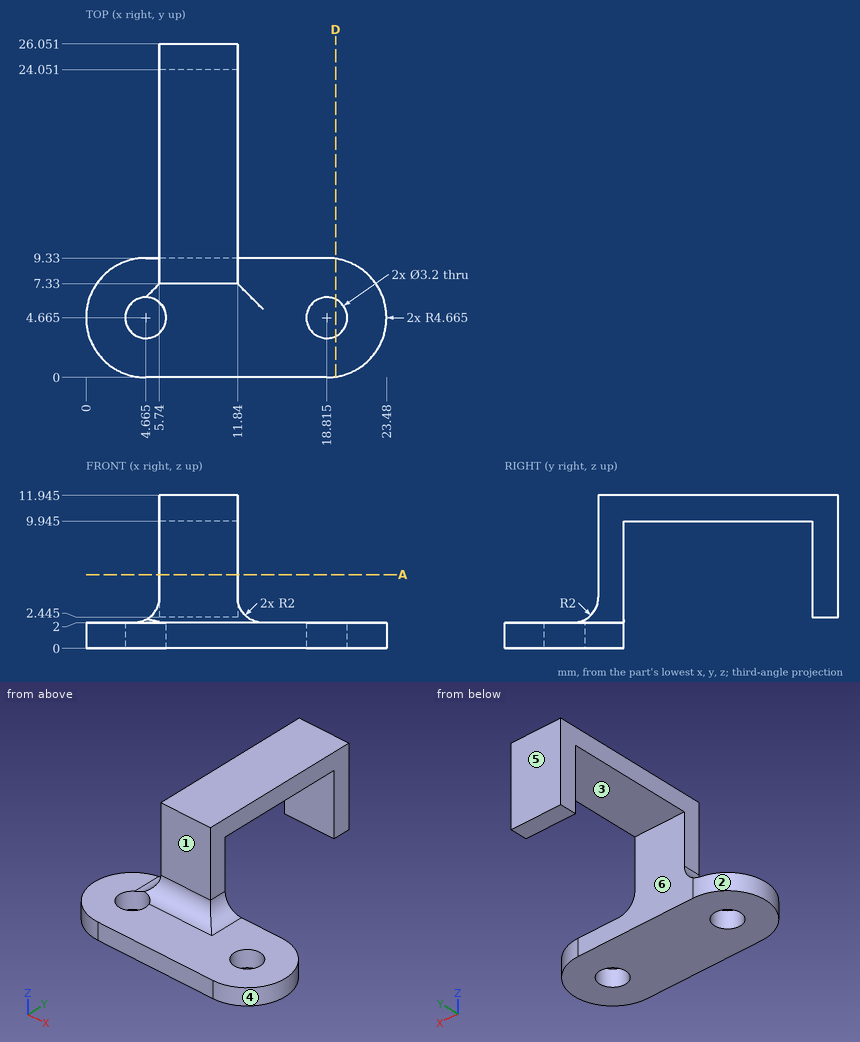
The drawing under review shows one solid part. Ordinate dimensions are in mm from its lowest x, y, z. A direction names the side the tool comes from. Give positions to 0.01 mm unless a question says otherwise; leave off trailing zeros. Write each loop counter-clockwise with the first axis right and the second up, starting at its lowest first coordinate (ties: lowest second). Pieces come first, ordered by that corner, then holes. Notation, with made-up numbers: (28, 42) -> (59, 42) arc R26 cw to (59, 62) -> close; hole circle Ø10 at (-17.75, 86). An arc over 180 degrees is marked (long way). Put each result on its own line as item: value.
(1) We need section D-D, the plane x = 19.5. Give the boundary of the cut face in (y, z), and give its area (3 significant figures).
Results are:
outline: (0.05, 0) -> (3.22, 0) -> (3.22, 2) -> (0.05, 2) -> close; (6.11, 0) -> (9.28, 0) -> (9.28, 2) -> (6.11, 2) -> close
area: 12.7 mm²
(2) We need section A-A, the plane z = 5.75. Give the boundary of the cut face in (x, y).
Results are:
outline: (5.74, 7.33) -> (11.84, 7.33) -> (11.84, 9.33) -> (5.74, 9.33) -> close; (5.74, 24.05) -> (11.84, 24.05) -> (11.84, 26.05) -> (5.74, 26.05) -> close
(3) The part is to be moulded in two halves that separate along Y. For the marked faces 4, 5 and 6, say which applies: pulls with the +Y half, pulls with the -Y half, needs draft (parallel to the pull), parting line crosses it, or undercut.
Results are:
face 4: parting line crosses it
face 5: pulls with the +Y half
face 6: undercut
(4) Tool access review of the marked faces 1, 2 and 3: name each direction out of +Z, -Z, +X, -X, +Y, -Y from which nothing blocks a thin tool from reaching the whole face with its end or side.
Results are:
face 1: +Z, +X, -X, -Y
face 2: +Z, -Z, -X
face 3: -Z, +X, -X
(5) To check wall thickness, follow probe 1 along Y at (x, z) = (7.75, 5.25); probe 2 along Y at (x, z) = (15.25, 1); probe 3 along X at (y, z) = (9.25, 5.5). State the ranges of each line that lie inside material, in increasing order. Write a range as from..to.
Results are:
probe 1: 7.33..9.33, 24.05..26.05
probe 2: 0..9.33
probe 3: 5.74..11.84
(6) For pin 1 Ø1.8 at (x, z) = (9, 6) entering from -Y; pin 2 Ø5 at (x, y) = (9.5, 14.5) entering from -Z (1 decimal); pin 3 Ø2 at (x, y) = (10, 25.5) entering from -Z (1 decimal), all flat-tipped, find the tip position at first contact; note any pin that passes through.
Results are:
pin 1: y = 7.33
pin 2: z = 9.9
pin 3: z = 2.4
